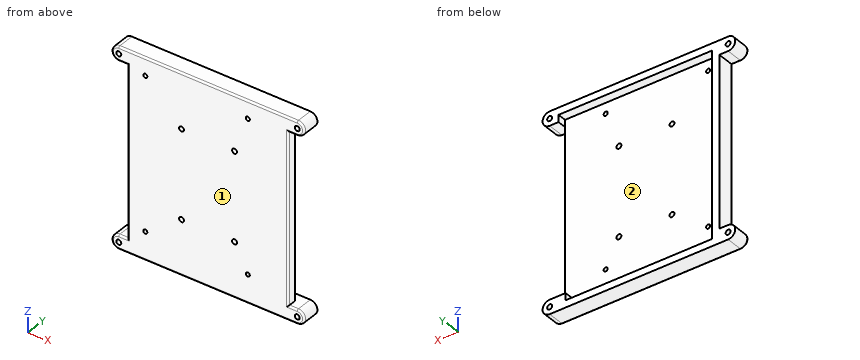
from build123d import *

# Parameters (mm, degrees)
SKETCH1_W                         = 91
SKETCH1_H                         = 112
SKETCH1_R                         = 1.15
BASE_DEPTH                        = 10
SKETCH2_W                         = 83
SKETCH2_H                         = 104
MODULE_CUTOUT_DEPTH               = 5
SKETCH3_R                         = 1.4
CASE_ASSEMBLY_HOLES_DEPTH         = 10
SKETCH5_W                         = 4
SKETCH5_H                         = 100
PORTS_SIDE_RECESS_DEPTH           = 5
BASKET_CLAMP_MOUNTING_HOLES_REACH = 80.78
SKETCH4_R                         = 1.4
F_1MM_EDGE_FILLETS_R              = 1


with BuildPart() as part:
    # Sketch1 → Base (new body)
    with BuildSketch(Plane(origin=(0, 0, 0), x_dir=(1, 0, 0), z_dir=(0, 1, 0))):
        Rectangle(SKETCH1_W, SKETCH1_H)
        with Locations(Location((-35.5, -46, 0), (0, 0, 270))):
            Circle(SKETCH1_R, mode=Mode.SUBTRACT)
        with Locations(Location((22.5, -46, 0), (0, 0, 270))):
            Circle(SKETCH1_R, mode=Mode.SUBTRACT)
        with Locations(Location((22.5, 40, 0), (0, 0, 270))):
            Circle(SKETCH1_R, mode=Mode.SUBTRACT)
        with Locations(Location((-35.5, 40, 0), (0, 0, 270))):
            Circle(SKETCH1_R, mode=Mode.SUBTRACT)
    extrude(amount=BASE_DEPTH)

    # Sketch2 → Module Cutout (cut)
    with BuildSketch(Plane(origin=(0, 10, 0), x_dir=(1, 0, 0), z_dir=(0, 1, 0))):
        Rectangle(SKETCH2_W, SKETCH2_H)
    extrude(amount=-MODULE_CUTOUT_DEPTH, mode=Mode.SUBTRACT)

    # Sketch3 → Case Assembly Holes (add)
    # profile 1 of 4: a face of its own
    with BuildSketch(Plane(origin=(0, 10, 0), x_dir=(1, 0, 0), z_dir=(0, 1, 0))):
        with BuildLine():
            Line((-45.5, 56), (-50.5, 56))
            ThreePointArc((-50.5, 56), (-54.5, 52), (-50.5, 48))
            Line((-50.5, 48), (-45.5, 48))
            Line((-45.5, 48), (-45.5, 56))
        make_face()
        with Locations(Location((-50.5, 52, 0), (0, 0, 270))):
            Circle(SKETCH3_R, mode=Mode.SUBTRACT)
    # profile 2 of 4: a face of its own
    with BuildSketch(Plane(origin=(0, 10, 0), x_dir=(1, 0, 0), z_dir=(0, 1, 0))):
        with BuildLine():
            Line((45.5, 48), (50.5, 48))
            ThreePointArc((50.5, 48), (54.5, 52), (50.5, 56))
            Line((50.5, 56), (45.5, 56))
            Line((45.5, 56), (45.5, 48))
        make_face()
        with Locations(Location((50.5, 52, 0), (0, 0, 270))):
            Circle(SKETCH3_R, mode=Mode.SUBTRACT)
    # profile 3 of 4: a face of its own
    with BuildSketch(Plane(origin=(0, 10, 0), x_dir=(1, 0, 0), z_dir=(0, 1, 0))):
        with BuildLine():
            Line((45.5, -56), (50.5, -56))
            ThreePointArc((50.5, -56), (54.5, -52), (50.5, -48))
            Line((50.5, -48), (45.5, -48))
            Line((45.5, -48), (45.5, -56))
        make_face()
        with Locations(Location((50.5, -52, 0), (0, 0, 270))):
            Circle(SKETCH3_R, mode=Mode.SUBTRACT)
    # profile 4 of 4: a face of its own
    with BuildSketch(Plane(origin=(0, 10, 0), x_dir=(1, 0, 0), z_dir=(0, 1, 0))):
        with BuildLine():
            Line((-45.5, -48), (-50.5, -48))
            ThreePointArc((-50.5, -48), (-54.5, -52), (-50.5, -56))
            Line((-50.5, -56), (-45.5, -56))
            Line((-45.5, -56), (-45.5, -48))
        make_face()
        with Locations(Location((-50.5, -52, 0), (0, 0, 270))):
            Circle(SKETCH3_R, mode=Mode.SUBTRACT)
    extrude(amount=-CASE_ASSEMBLY_HOLES_DEPTH)

    # Sketch5 → Ports Side Recess (cut)
    with BuildSketch(Plane(origin=(0, 10, 0), x_dir=(1, 0, 0), z_dir=(0, 1, 0))):
        with Locations((43.5, -2)):
            Rectangle(SKETCH5_W, SKETCH5_H)
    extrude(amount=-PORTS_SIDE_RECESS_DEPTH, mode=Mode.SUBTRACT)

    # Sketch4 → Basket Clamp Mounting Holes (cut, up to next)
    with BuildSketch(Plane.XZ, mode=Mode.PRIVATE) as basket_clamp_mounting_holes_sk1:
        with Locations(Location((-15, 25, 0), (0, 0, 270))):
            Circle(SKETCH4_R)
    basket_clamp_mounting_holes_tool1 = extrude(basket_clamp_mounting_holes_sk1.sketch, amount=-BASKET_CLAMP_MOUNTING_HOLES_REACH, mode=Mode.PRIVATE) & part.part
    # Sketch4 → Basket Clamp Mounting Holes (cut, up to next)
    with BuildSketch(Plane.XZ, mode=Mode.PRIVATE) as basket_clamp_mounting_holes_sk2:
        with Locations(Location((-15, -25, 0), (0, 0, 270))):
            Circle(SKETCH4_R)
    basket_clamp_mounting_holes_tool2 = extrude(basket_clamp_mounting_holes_sk2.sketch, amount=-BASKET_CLAMP_MOUNTING_HOLES_REACH, mode=Mode.PRIVATE) & part.part
    # Sketch4 → Basket Clamp Mounting Holes (cut, up to next)
    with BuildSketch(Plane.XZ, mode=Mode.PRIVATE) as basket_clamp_mounting_holes_sk3:
        with Locations(Location((15, -25, 0), (0, 0, 270))):
            Circle(SKETCH4_R)
    basket_clamp_mounting_holes_tool3 = extrude(basket_clamp_mounting_holes_sk3.sketch, amount=-BASKET_CLAMP_MOUNTING_HOLES_REACH, mode=Mode.PRIVATE) & part.part
    # Sketch4 → Basket Clamp Mounting Holes (cut, up to next)
    with BuildSketch(Plane.XZ, mode=Mode.PRIVATE) as basket_clamp_mounting_holes_sk4:
        with Locations(Location((15, 25, 0), (0, 0, 270))):
            Circle(SKETCH4_R)
    basket_clamp_mounting_holes_tool4 = extrude(basket_clamp_mounting_holes_sk4.sketch, amount=-BASKET_CLAMP_MOUNTING_HOLES_REACH, mode=Mode.PRIVATE) & part.part
    add(basket_clamp_mounting_holes_tool1.solids().sort_by_distance((-15, 0, 25))[0], mode=Mode.SUBTRACT)
    add(basket_clamp_mounting_holes_tool2.solids().sort_by_distance((-15, 0, -25))[0], mode=Mode.SUBTRACT)
    add(basket_clamp_mounting_holes_tool3.solids().sort_by_distance((15, 0, -25))[0], mode=Mode.SUBTRACT)
    add(basket_clamp_mounting_holes_tool4.solids().sort_by_distance((15, 0, 25))[0], mode=Mode.SUBTRACT)

    # 1mm Edge Fillets
    f_1mm_edge_fillets_edges = [part.edges().sort_by_distance(p)[0] for p in [
        (0, 0, -56),
        (-45.5, 0, 0),
        (-48, 0, -48),
        (-54.5, 0, -52),
        (0, 0, 56),
        (54.5, 0, -52),
        (48, 0, -48),
        (45.5, 0, 0),
        (54.5, 0, 52),
        (48, 0, 48),
        (-54.5, 0, 52),
        (-48, 0, 48),
    ]]
    fillet(f_1mm_edge_fillets_edges, radius=F_1MM_EDGE_FILLETS_R)


solid = part.part
Work out the finished part from the listing and answer in its coordinate system (mm). Face numbers are marked on the shaded views. Round coordinates to 2 decimals unless told otherwise and drop trailing zeros. Loops run counter-clockwise (first coordinate to the right, second up) from the corner with the lowest first, then second, coordinate; pieces in that order, holes last. Notation, with made-up numbers: (80, 12) -> (122, 12) arc R6 ccw to (122, 23) -> close; hole circle Ø1 at (61, 51). An arc over 180 degrees is marked (long way). Use one line per item in the form item = value.
(1) Straight lines are drawn through the part: line 1 (Z direction, x = 22.5, y = 2.05); line 2 (Z direction, x = -21.5, y = 5.75); line 3 (X direction, y = 2.6, z = -40). For each, find the intervals that lie inside material, in ascending order.
Answer list:
line_1 = -56 to -41.15, -38.85 to 44.85, 47.15 to 56
line_2 = -56 to -52, 52 to 56
line_3 = -45.5 to -36.65, -34.35 to 21.35, 23.65 to 45.5
(2) Find section A-A on x = 15. Give the vertices of the cut face in (y, z), then the cut area to 3 significant figures.
Answer list:
outline = (0, -55) arc R1 ccw to (1, -56) -> (10, -56) -> (10, -52) -> (5, -52) -> (5, -26.4) -> (0, -26.4) -> close; (0, -23.6) -> (5, -23.6) -> (5, 23.6) -> (0, 23.6) -> close; (0, 26.4) -> (5, 26.4) -> (5, 52) -> (10, 52) -> (10, 56) -> (1, 56) arc R1 ccw to (0, 55) -> close
area = 572 mm2
(3) Find section C-C on z = 31.5. Give the vertices of the cut face in (x, y), then the cut area to 3 significant figures.
Answer list:
outline = (-45.5, 1) arc R1 ccw to (-44.5, 0) -> (44.5, 0) arc R1 ccw to (45.5, 1) -> (45.5, 5) -> (-41.5, 5) -> (-41.5, 10) -> (-45.5, 10) -> close
area = 475 mm2
(4) Flat-ended cylindrical pins translate along their axes: P1, Ø6, axis at y = 1.5, z = 7, coming from the -X side; P2, Ø2, axis at y = 5, z = 31, coming from the +X side; P3, Ø2, axis at x = 22.5, z = -40, coming from the +Y side; P4, Ø3.5, axis at x = -15, z = -25, coming from the +Y side. Find the tip coordinate at first contact, or state that the pin passes through.
Answer list:
P1 = -45.5
P2 = 45.5
P3 = through
P4 = 5
(5) Find section B-B on z = -25. Give the vertices of the cut face in (x, y), then the cut area to 3 significant figures.
Answer list:
outline = (-45.5, 1) arc R1 ccw to (-44.5, 0) -> (-16.4, 0) -> (-16.4, 5) -> (-41.5, 5) -> (-41.5, 10) -> (-45.5, 10) -> close; (-13.6, 0) -> (13.6, 0) -> (13.6, 5) -> (-13.6, 5) -> close; (16.4, 0) -> (44.5, 0) arc R1 ccw to (45.5, 1) -> (45.5, 5) -> (16.4, 5) -> close
area = 447 mm2
(6) For a pull along Z with two mould halves and no side action, classify the marked faces 1 and 2 as released by +Z, released by -Z, zero draft, split by the parting line, or undercut.
Answer list:
face_1 = zero draft
face_2 = undercut
